Verification items for the finished model (mm, model axes). A direction names the side the tool comes from. Round coordinates to 2 decimals unless told otherwise and drop trailing zeros. Order: outer loops, then holes, each group sorted by start corner. A loop starts at its lowest first (then second) coordinate and runs counter-clockwise, first axis right, second up.
```python
from build123d import *

# Parameters (mm, degrees)
F2_R     = 4
F3_DEPTH = 2
F4_SIZE  = 0.5


with BuildPart() as f1:
    # F0 (on Front) → F1 (revolve)
    with BuildSketch(Plane.XZ):
        Polygon((0, 15), (0, 0), (10, 0), (10, 7), (7, 11), (7, 15), align=None)
    revolve(axis=Axis((0, 0, 7.5), (0, 0, -1)))

    # F2 (on face) → F3 (cut)
    with BuildSketch(Plane.XY.offset(15)):
        Circle(F2_R)
    extrude(amount=-F3_DEPTH, mode=Mode.SUBTRACT)

    # F4
    f4_edges = [f1.edges().sort_by_distance(p)[0] for p in [
        (-10, 0, 0),
    ]]
    chamfer(f4_edges, length=F4_SIZE)


solid = f1.part
```
1) Tool access check on faces 1 (the cylindrical face through (-2.17, 9.76, 3.8)), 2 (the cylindrical face through (6.466, 2.681, 13.028)). Record the directions out of +Z, -Z, +X, -X, +Y, -Y that give a thin tool (end or side, any length) a straight path to the whole face; none if there is none.
2) Sectioned sample at A-A on x = 0. Record the cut outline in (y, z).
3) Draft check along Y on faces 3 (the cylindrical face through (-0.867, -3.905, 14.014)), 4 (the conical face through (-5.671, 4.348, 10.806)), 5 (the flat face through (0, 0, 0)). Enter one of: released by +Y, released by -Y, zero draft, split by the parting line, or undercut.
4) Scan lines: probe 1 along Y at (x, z) = (0, 14.15); probe 2 along Y at (x, z) = (-2.25, 14); probe 3 along Z at (x, y) = (0.75, 0.75). Record each from-to range of solid material in increasing order.
5) Go/stop test with flat-tipped pins: pin 1 Ø1.5 at (y, z) = (-2, 6.5) entering from -X; pin 2 Ø4 at (x, y) = (-1.5, 0.5) entering from +Z; pin 3 Ø1 at (y, z) = (-2.5, 4) entering from -X. Record where each tip stops, or that it passes through.
Returned:
1. face 1: +Z, -Z
1. face 2: +Z
2. outline: (-10, 0.5) - (-9.5, 0) - (9.5, 0) - (10, 0.5) - (10, 7) - (7, 11) - (7, 15) - (4, 15) - (4, 13) - (-4, 13) - (-4, 15) - (-7, 15) - (-7, 11) - (-10, 7) - close
3. face 3: undercut
3. face 4: split by the parting line
3. face 5: zero draft
4. probe 1: y = -7 to -4, 4 to 7
4. probe 2: y = -6.63 to -3.31, 3.31 to 6.63
4. probe 3: z = 0 to 13
5. pin 1: stops at x = -9.92
5. pin 2: stops at z = 13
5. pin 3: stops at x = -9.8
